```python
from build123d import *

# Parameters (mm, degrees)
SKETCH1_R           = 40
SKETCH1_R_2         = 1.5
BOSS_EXTRUDE1_DEPTH = 4


with BuildPart() as part:
    # Sketch1 → Boss-Extrude1 (new body)
    with BuildSketch(Plane(origin=(0, 0, 0), x_dir=(1, 0, 0), z_dir=(0, 1, 0))):
        with Locations(Location((0, 0, 0), (0, 0, 270))):
            Circle(SKETCH1_R)
        with Locations(Location((0, -12.5, 0), (0, 0, 270))):
            Circle(SKETCH1_R_2, mode=Mode.SUBTRACT)
        with Locations(Location((-12.5, 0, 0), (0, 0, 270))):
            Circle(SKETCH1_R_2, mode=Mode.SUBTRACT)
        with Locations(Location((0, 12.5, 0), (0, 0, 270))):
            Circle(SKETCH1_R_2, mode=Mode.SUBTRACT)
        with Locations(Location((12.5, 0, 0), (0, 0, 270))):
            Circle(SKETCH1_R_2, mode=Mode.SUBTRACT)
        with BuildLine():
            ThreePointArc((23.783141558, 28.343644395), (20.965477453, 28.097130729), (21.21199112, 25.279466623))
            ThreePointArc((21.21199112, 25.279466623), (31.009856486, -11.28666473), (0, -33))
            ThreePointArc((0, -33), (-2, -35), (0, -37))
            ThreePointArc((0, -37), (34.768626969, -12.654745303), (23.783141558, 28.343644395))
        make_face(mode=Mode.SUBTRACT)
    extrude(amount=BOSS_EXTRUDE1_DEPTH)


solid = part.part
```
Input: part model. Units: mm. Frame: model coordinates. A direction names the side the tool comes from. Coordinates: 2 decimals unless noted, no trailing zeros. Write each loop counter-clockwise with the first axis right and the second up, starting at its lowest first coordinate (ties: lowest second). Pieces come first, ordered by that corner, then holes. Notation, with made-up numbers: (75, -38.75) -> (96, -38.75) arc R19 ccw to (96, -18.75) -> close; hole circle Ø7 at (-8, -4.75). An arc over 180 degrees is marked (long way). Answer as a JSON object with one key per item and string values.
1. Section A-A on z = 0. Return the cut outline in (x, y).
Result set:
{"outline": "(-40, 0) -> (-14, 0) -> (-14, 4) -> (-40, 4) -> close; (-11, 0) -> (11, 0) -> (11, 4) -> (-11, 4) -> close; (14, 0) -> (33, 0) -> (33, 4) -> (14, 4) -> close; (37, 0) -> (40, 0) -> (40, 4) -> (37, 4) -> close"}
2. Section C-C on z = 35. Return the cut outline in (x, y).
Result set:
{"outline": "(-19.36, 0) -> (-2, 0) -> (-2, 4) -> (-19.36, 4) -> close; (12, 0) -> (19.36, 0) -> (19.36, 4) -> (12, 4) -> close"}
3. First-contact query: P1, Ø2, axis at y = 1, z = 6.5, coming from the -X side; P2, Ø1.5, axis at y = 3, z = 2, coming from the +X side. Flat tips, straight axial feed; report the tip coordinate or a pass-through.
Result set:
{"P1": "stops at x = -39.62", "P2": "stops at x = 39.98"}
4. Material intervals for line 1 (X direction, y = 2.7, z = 0); line 2 (Z direction, x = 13.5, y = 3.65); line 3 (X direction, y = 1.7, z = 12.5), sorted ascending. Write a range as from..to.
Result set:
{"line 1": "x = -40..-14, -11..11, 14..33, 37..40", "line 2": "z = -37.65..-1.12, 1.12..30.11, 34.45..37.65", "line 3": "x = -38..-1.5, 1.5..30.54, 34.82..38"}
5. Mould query, pull axis Z, two halves, no side actions, for faces 3 (the face through (1, 0, -1)), 4 (the face through (-39.05, 1.97, -8.67)), 5 (the face through (20.994, 1.972, -28.131)). Classes: released by +Z, released by -Z, zero draft, split by the parting line, or undercut.
Result set:
{"face 3": "zero draft", "face 4": "split by the parting line", "face 5": "undercut"}
6. Access query for faces 1 (the face through (1, 4, -1)), 2 (the face through (31.2, 1.97, 10.75)). Directions: +Z, -Z, +X, -X, +Y, -Y. A direction counts if a zero-diameter tool reaches every point of the face in a straight line with its end or side. Return the directions, or none.
Result set:
{"face 1": "+Z, -Z, +X, -X, +Y", "face 2": "+Y, -Y"}
7. Section B-B on x = -12.5. Return the cut outline in (y, z), then the cut area to 3 significant figures.
Result set:
{"outline": "(0, -38) -> (4, -38) -> (4, -1.5) -> (0, -1.5) -> close; (0, 1.5) -> (4, 1.5) -> (4, 38) -> (0, 38) -> close", "area": "292 mm2"}
8. Section D-D on z = -12. Return the cut outline in (x, y), then the cut area to 3 significant figures.
Result set:
{"outline": "(-38.16, 0) -> (-1.41, 0) -> (-1.41, 4) -> (-38.16, 4) -> close; (1.41, 0) -> (30.74, 0) -> (30.74, 4) -> (1.41, 4) -> close; (35, 0) -> (38.16, 0) -> (38.16, 4) -> (35, 4) -> close", "area": "277 mm2"}
